```python
from build123d import *

# Parameters (mm, degrees)
F0_R            = 75
F1_DEPTH        = 3
F3_DEPTH        = 3
F3_COPIES_COUNT = 12


# Not quite as in the source:
# - a pattern or mirror of a feature is missing from the dataset's text; its kind, count and spacing are read off the source's solid


with BuildPart() as f1:
    # F0 (on Top) → F1 (new body)
    with BuildSketch(Plane.XY):
        Circle(F0_R)
    extrude(amount=F1_DEPTH)

    # F2 (on Top) → F3 (cut, through all)
    with BuildSketch(Plane.XY):
        with BuildLine():
            Line((23.905803232, 71.0880620909), (28.1729654475, 73.6940794788))
            Line((28.1729654475, 73.6940794788), (19.7568770352, 72.3509903859))
            ThreePointArc((19.7568770352, 72.3509903859), (21.840470668, 71.7495215385), (23.905803232, 71.0880620909))
        make_face()
        with BuildLine():
            Line((11.1043165854, 63.2700099269), (23.905803232, 71.0880620909))
            ThreePointArc((23.905803232, 71.0880620909), (21.840470668, 71.7495215385), (19.7568770352, 72.3509903859))
            Line((19.7568770352, 72.3509903859), (9.5407061526, 65.8303072562))
            Line((9.5407061526, 65.8303072562), (11.1043165854, 63.2700099269))
        make_face()
    f3 = extrude(amount=F3_DEPTH, mode=Mode.SUBTRACT)

    # F3_copies: F3 ×12 about axis
    f3_copies_axis = Axis((0, 0, 0), (0, 0, 1))
    for i in range(1, F3_COPIES_COUNT):
        add(f3.rotate(f3_copies_axis, i * 360 / F3_COPIES_COUNT), mode=Mode.SUBTRACT)


solid = f1.part
```
Here's how the part is built. I have some questions about the finished solid (model axes, mm). A direction names the side the tool comes from. Give positions to 0.01 mm unless a question says otherwise; leave off trailing zeros. Write each loop counter-clockwise with the first axis right and the second up, starting at its lowest first coordinate (ties: lowest second). Pieces come first, ordered by that corner, then holes. Notation, with made-up numbers: (6.5, -9) -> (37.5, -9) arc R22 ccw to (37.5, 9) -> close; hole circle Ø11 at (10, -3.75). An arc over 180 degrees is marked (long way). Use one line per item in the form item = value.
1) Suppose I cut it at B-B (x = 17). Please give me the cut outline in (y, z), and give its area (3 significant figures).
Verdict:
outline = (-69.55, 0) -> (66.87, 0) -> (66.87, 3) -> (-69.55, 3) -> close; (70.59, 0) -> (73.05, 0) -> (73.05, 3) -> (70.59, 3) -> close
area = 417 mm2
2) We'd pull the mould along Y, two halves only. Please class faces 1 (the face through (63.522, -39.874, 1.479)), 2 (the face through (-1, 1, 0)), 3 (the face through (-17.415, -67.124, 1.479)), 4 (the face through (17.415, 67.124, 1.479)): +Y half, -Y half, draft (parallel to the pull), parting line (faces both ways), or undercut.
Verdict:
face_1 = -Y half
face_2 = draft
face_3 = undercut
face_4 = undercut
3) Suppose I cut it at C-C (y = -36). Please give me the cut outline in (x, z), and give its area (3 significant figures).
Verdict:
outline = (-65.8, 0) -> (65.8, 0) -> (65.8, 3) -> (-65.8, 3) -> close
area = 395 mm2
4) If I drill on L1, parallel to Y at x = 19.5, z = 0.55; L2, parallel to X at y = 48, z = 1.4; L3, parallel to X at y = -50, z = 2.8, over which ranges is the centre line in solid material (lowest first)? Write a range as [from, to].
Verdict:
L1 = [-72.42, -71.7], [-64.97, 68.4], [72.19, 72.42]
L2 = [-57.63, -52.54], [-49.41, 57.63]
L3 = [-41.23, 49.46], [52.63, 55.9]
5) Suppose I cut it at A-A (y = 46). Please give me the cut outline in (x, z).
Verdict:
outline = (-59.24, 0) -> (-52.46, 0) -> (-52.46, 3) -> (-59.24, 3) -> close; (-49.36, 0) -> (59.24, 0) -> (59.24, 3) -> (-49.36, 3) -> close
6) I'm going to push flat-ended pins straight in: pin 1 (1.5 mm diameter, centred on y = -9, z = 1.5, fed in from -X); pin 2 (1 mm diameter, centred on x = 36.5, z = 1, fed in from +Y). Where does each tip first touch, or does it pass through?
Verdict:
pin_1 = -74.54
pin_2 = 65.8
7) On a 3-axis mill with a long thin cutter (end or side, diameter ignored), from which of +Z, -Z, +X, -X, +Y, -Y can I reach the whole of each face in a straight line? I mean faces 5 (the face through (-21.82, 67.23, 1.48)), 6 (the face through (-63.522, 39.874, 1.479)). Say none if no direction works.
Verdict:
face_5 = +Z, -Z
face_6 = +Z, -Z, -X, +Y
